Check sheet for the modelled part. Datum: model origin and axes. Units: mm. Round coordinates to 2 decimals unless told otherwise and drop trailing zeros. Loops run counter-clockwise (first coordinate to the right, second up) from the corner with the lowest first, then second, coordinate; pieces in that order, holes last. Notation, with made-up numbers: (50.5, 54) - (88.5, 54) arc R21 cw to (88.5, 58) - close; hole circle Ø2 at (1, 89). An arc over 180 degrees is marked (long way). Put each result on its own line as item: value. Start each with the question number.
Item 1: Section check C-C, the plane y = -3. Record the cut outline in (x, z), and give its area (3 significant figures).
Item 2: Material ranges on line 1 along X through (y, z) = (-5.75, 0); line 2 along X through (y, z) = (-10.5, -1.25); line 3 along Z through (x, y) = (0.25, -8), recorded low to high.
Item 3: Section check B-B, the plane z = 0. Record the cut outline in (x, y), and give its area (3 significant figures).
Item 4: Section check A-A, the plane x = 0. Record the cut outline in (y, z).
Item 5: Draft check along Z on faces 1 (the cylindrical face through (3.778, -6.265, -0.496)), 2 (the cylindrical face through (0.354, -6.435, 1.593)), 3 (the flat face through (-2, 0, 2)). Enter one of: pulls with the +Z half, pulls with the -Z half, needs draft (parallel to the pull), parting line crosses it, or undercut.
from build123d import *

# Parameters (mm, degrees)
SKETCH1_R                    = 3.81
BOSS_EXTRUDE1_DEPTH          = 12.7
F_30_0_1285_DIAMETER_HOLE1_D = 3.2639
CHAMFER1_SIZE                = 0.254


with BuildPart() as part:
    # Sketch1 → Boss-Extrude1 (new body)
    with BuildSketch(Plane(origin=(0, 0, 0), x_dir=(1, 0, 0), z_dir=(0, 1, 0))):
        with Locations(Location((0, 0, 0), (0, 0, 270))):
            Circle(SKETCH1_R)
    extrude(amount=-BOSS_EXTRUDE1_DEPTH)

    # #30 (0.1285) Diameter Hole1 (through all)
    with Locations(Plane(origin=(0, 0, 0), x_dir=(1, 0, 0), z_dir=(0, 1, 0))):
        with Locations((0, 0)):
            Hole(F_30_0_1285_DIAMETER_HOLE1_D / 2)

    # Chamfer1
    chamfer1_edges = [part.edges().sort_by_distance(p)[0] for p in [
        (0, 0, -3.81),
        (0, -12.7, -3.81),
        (1.63195, 0, 0),
        (1.63195, -12.7, 0),
    ]]
    chamfer(chamfer1_edges, length=CHAMFER1_SIZE)


solid = part.part
Check result:
1. outline: circle Ø7.62 at (0, 0); hole circle Ø3.26 at (0, 0)
1. area: 37.2 mm²
2. line 1: -3.81 to -1.63, 1.63 to 3.81
2. line 2: -3.6 to -1.05, 1.05 to 3.6
2. line 3: -3.8 to -1.61, 1.61 to 3.8
3. outline: (-3.81, -12.45) - (-3.56, -12.7) - (-1.89, -12.7) - (-1.63, -12.45) - (-1.63, -0.25) - (-1.89, 0) - (-3.56, 0) - (-3.81, -0.25) - close; (1.63, -12.45) - (1.89, -12.7) - (3.56, -12.7) - (3.81, -12.45) - (3.81, -0.25) - (3.56, 0) - (1.89, 0) - (1.63, -0.25) - close
3. area: 55.1 mm²
4. outline: (-12.7, -3.56) - (-12.45, -3.81) - (-0.25, -3.81) - (0, -3.56) - (0, -1.89) - (-0.25, -1.63) - (-12.45, -1.63) - (-12.7, -1.89) - close; (-12.7, 1.89) - (-12.45, 1.63) - (-0.25, 1.63) - (0, 1.89) - (0, 3.56) - (-0.25, 3.81) - (-12.45, 3.81) - (-12.7, 3.56) - close
5. face 1: parting line crosses it
5. face 2: undercut
5. face 3: needs draft
